For this review, take the finished solid that the model builds, in its own axes (mm). Face numbers are marked on the shaded views. Coordinates: 2 decimals unless noted, no trailing zeros. Order: outer loops, then holes, each group sorted by start corner. A loop starts at its lowest first (then second) coordinate and runs counter-clockwise, first axis right, second up. Notation, with made-up numbers: (-19.5, 37) -> (0.5, 37) arc R29 cw to (0.5, 67) -> close; hole circle Ø5 at (64, 82). An arc over 180 degrees is marked (long way). Write item = value, one per line. Start each with the question number.
1) Draft analysis for pull direction Y (two halves, no side actions). For the marked faces 1, 2 and 3, state which applies: +Y half, -Y half, draft (parallel to the pull), parting line (faces both ways), or undercut.
2) Wall thickness on probe 1 along Y at (x, z) = (2.25, 4.75); probe 2 along Y at (x, z) = (0, 9); probe 3 along Z at (x, y) = (2.75, 27) (3 decimals): over which ranges is each line inside the solid? List them lowest first. Write a range as [from, to].
3) Consider section C-C on y = 26. Give the boundary of the cut face in (x, z) (1 decimal).
4) Consider section A-A on z = 4. State how many separate pieces and enclosed holes the cut face has, and give its area (3 significant figures).
5) Insertion check: pin 1 Ø0.7 at (x, y) = (0, -15.5) entering from +Z (3 decimals); pin 2 Ø5.5 at (y, z) = (-26.99, 4.76) entering from +X. Each pin has a flat end and moves straight along its axis. Give the tip position at first contact, or say it passes through.
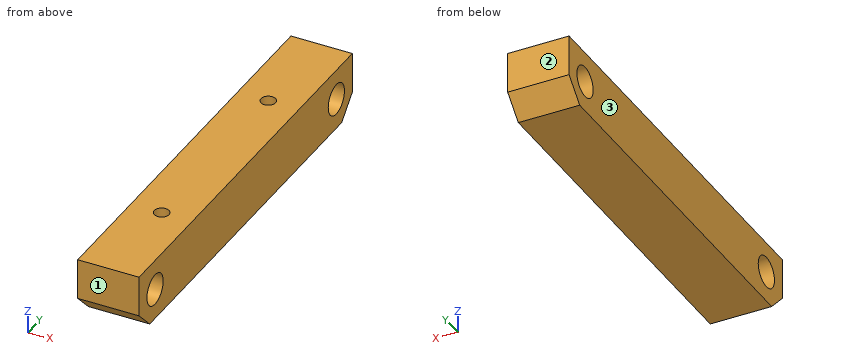
from build123d import *

# Parameters (mm, degrees)
F0_W     = 9.525
F0_H     = 63.5
F1_DEPTH = 9.525
F2_R     = 2.413
F3_DEPTH = 9.526
F4_R     = 1.143
F5_DEPTH = 6.35
F6_SIZE  = 3.175


# Not quite as in the source:
# - a pattern or mirror of a feature is missing from the dataset's text; its kind, count and spacing are read off the source's solid


with BuildPart() as f1:
    # F0 (on Top) → F1 (new body)
    with BuildSketch(Plane.XY):
        Rectangle(F0_W, F0_H)
    extrude(amount=F1_DEPTH)

    # F2 (on face) → F3 (cut, through all)
    with BuildSketch(Plane.YZ.offset(4.7625)):
        with Locations((-26.9875, 4.7625)):
            Circle(F2_R)
    f3 = extrude(amount=-F3_DEPTH, mode=Mode.SUBTRACT)

    # F3_copies: F3 across plane
    add(f3.mirror(Plane.ZX), mode=Mode.SUBTRACT)

    # F4 (on face) → F5 (cut)
    with BuildSketch(Plane.XY.offset(9.525)):
        with Locations((0, 15.875)):
            Circle(F4_R)
    f5 = extrude(amount=-F5_DEPTH, mode=Mode.SUBTRACT)

    # F5_copies: F5 across plane
    add(f5.mirror(Plane(origin=(0, 0, 0), x_dir=(0, 0, -1), z_dir=(0, -1, 0))), mode=Mode.SUBTRACT)

    # F6
    f6_edges = [f1.edges().sort_by_distance(p)[0] for p in [
        (0, -31.75, 0),
        (0, 31.75, 0),
    ]]
    chamfer(f6_edges, length=F6_SIZE)


solid = f1.part
Answer sheet:
q1.face_1 = -Y half
q1.face_2 = +Y half
q1.face_3 = draft
q2.probe_1 = [-31.75, -29.4], [-24.57, 24.57], [29.4, 31.75]
q2.probe_2 = [-31.75, -17.02], [-14.73, 14.73], [17.02, 31.75]
q2.probe_3 = [0, 2.35], [7.175, 9.525]
q3.outline = (-4.8, 0) -> (4.8, 0) -> (4.8, 2.6) -> (-4.8, 2.6) -> close; (-4.8, 7) -> (4.8, 7) -> (4.8, 9.5) -> (-4.8, 9.5) -> close
q4.separate_pieces = 3
q4.enclosed_holes = 2
q4.area = 509 mm2
q5.pin_1 = 3.175
q5.pin_2 = 4.76
